Part model, mm, in its own coordinate system. A direction names the side the tool comes from. Give positions to 0.01 mm unless a question says otherwise; leave off trailing zeros. Loops run counter-clockwise (first coordinate to the right, second up) from the corner with the lowest first, then second, coordinate; pieces in that order, holes last. Notation, with made-up numbers: (62, -9.5) -> (100, -9.5) arc R27 ccw to (100, 11.5) -> close; hole circle Ø7 at (67, 3). An arc over 180 degrees is marked (long way). Write item = value, one per line.
from build123d import *

# Parameters (mm, degrees)
SKETCH1_R                      = 4.975
BOSS_EXTRUDE1_DEPTH            = 9.5
SKETCH2_R                      = 3
BOSS_EXTRUDE2_DEPTH            = 17
CUT_EXTRUDE1_REACH             = 6.975
SKETCH3_R                      = 0.465864979
CUT_EXTRUDE1_DIRECTION_2_REACH = 6.975
SKETCH5_W                      = 19.55
SKETCH5_H                      = 22.35
BOSS_EXTRUDE4_DEPTH            = 9.25


with BuildPart() as part:
    # Sketch1 → Boss-Extrude1 (new body)
    with BuildSketch(Plane.XY):
        Circle(SKETCH1_R)
    extrude(amount=BOSS_EXTRUDE1_DEPTH)

    # Sketch2 → Boss-Extrude2 (add)
    with BuildSketch(Plane.XY.offset(9.5)):
        Circle(SKETCH2_R)
    extrude(amount=BOSS_EXTRUDE2_DEPTH)

    # Sketch3 → Cut-Extrude1 (cut, up to next)
    with BuildSketch(Plane(origin=(0, 0, 0), x_dir=(1, 0, 0), z_dir=(0, 1, 0)), mode=Mode.PRIVATE) as cut_extrude1_sk1:
        with Locations((0, -23)):
            Circle(SKETCH3_R)
    cut_extrude1_tool1 = extrude(cut_extrude1_sk1.sketch, amount=-CUT_EXTRUDE1_REACH, mode=Mode.PRIVATE) & part.part
    add(cut_extrude1_tool1.solids().sort_by_distance((0, 0, 23))[0], mode=Mode.SUBTRACT)

    # Sketch3 → Cut-Extrude1 direction 2 (cut, up to next)
    with BuildSketch(Plane(origin=(0, 0, 0), x_dir=(1, 0, 0), z_dir=(0, 1, 0)), mode=Mode.PRIVATE) as cut_extrude1_direction_2_sk1:
        with Locations((0, -23)):
            Circle(SKETCH3_R)
    cut_extrude1_direction_2_tool1 = extrude(cut_extrude1_direction_2_sk1.sketch, amount=CUT_EXTRUDE1_DIRECTION_2_REACH, mode=Mode.PRIVATE) & part.part
    add(cut_extrude1_direction_2_tool1.solids().sort_by_distance((0, 0, 23))[0], mode=Mode.SUBTRACT)

    # Sketch5 → Boss-Extrude4 (add)
    with BuildSketch(Plane(origin=(0, 0, 0), x_dir=(-1, 0, 0), z_dir=(0, 0, -1))):
        Rectangle(SKETCH5_W, SKETCH5_H)
    extrude(amount=BOSS_EXTRUDE4_DEPTH)


solid = part.part
1) Slice it at C-C, the plane z = 21.5. List the corners of the cut face in (x, y), and give its area (3 significant figures).
Resolved:
outline = circle Ø6 at (0, 0)
area = 28.3 mm²
2) Slice it at A-A, the plane x = 0. List the corners of the cut face in (y, z) (3 decimals), and give its area (3 significant figures).
Resolved:
outline = (-11.175, -9.25) -> (11.175, -9.25) -> (11.175, 0) -> (4.975, 0) -> (4.975, 9.5) -> (3, 9.5) -> (3, 22.534) -> (-3, 22.534) -> (-3, 9.5) -> (-4.975, 9.5) -> (-4.975, 0) -> (-11.175, 0) -> close; (-3, 23.466) -> (3, 23.466) -> (3, 26.5) -> (-3, 26.5) -> close
area = 398 mm²
3) Drill centre lines: line 1 along Z through (x, y) = (0, -1.2); line 2 along Z through (x, y) = (6.25, -1.5); line 3 along X through (y, z) = (1.2, 23). Where is each one in solid material? Low to high. Write a range as [from, to].
Resolved:
line_1 = [-9.25, 22.53], [23.47, 26.5]
line_2 = [-9.25, 0]
line_3 = [-2.75, -0.47], [0.47, 2.75]
4) Which spindle directions (+Z, -Z, +X, -X, +Y, -Y) get a long thin tool onto all of the face, cutting with end or side? Do faces 1 (the face through (9.775, 0, -5)), 2 (the face through (4.5, 2.6, 0)). Say none if no direction does.
Resolved:
face_1 = +Z, -Z, +X, +Y, -Y
face_2 = +Z
5) Slice it at B-B, the plane y = -6.5. List the corners of the cut face in (x, z) (3 decimals).
Resolved:
outline = (-9.775, -9.25) -> (9.775, -9.25) -> (9.775, 0) -> (-9.775, 0) -> close
6) Drop flat-ended pins along their axis: P1, Ø1, axis at y = 4.5, z = 17.5, coming from the +X side; P2, Ø1, axis at x = -1.5, z = 11, coming from the -Y side; P3, Ø1.5, axis at y = 0, z = 16.5, coming from the -X side. Give the stop position or say it passes through.
Resolved:
P1 = through
P2 = -2.83
P3 = -3
7) Slice it at D-D, the plane x = -5.5. List the corners of the cut face in (y, z) (3 decimals), and give its area (3 significant figures).
Resolved:
outline = (-11.175, -9.25) -> (11.175, -9.25) -> (11.175, 0) -> (-11.175, 0) -> close
area = 207 mm²
